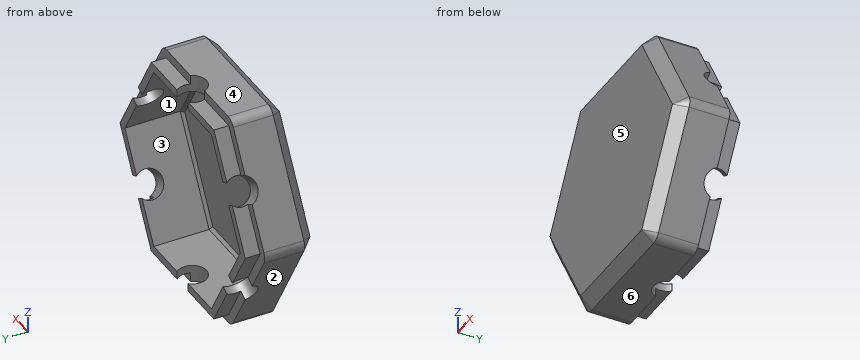
```python
from build123d import *

# Parameters (mm, degrees)
BOSS_EXTRUDE1_START = -3.7
BOSS_EXTRUDE1_DEPTH = 10
CUT_EXTRUDE1_DEPTH  = 8.6
BOSS_EXTRUDE2_DEPTH = 1.6
FILLET1_R           = 2
CUT_EXTRUDE4_DEPTH  = 1
CUT_EXTRUDE3_START  = -3
SKETCH4_R           = 2.5
CUT_EXTRUDE3_DEPTH  = 3
CIRPATTERN1_COUNT   = 6
CHAMFER1_SIZE       = 0.5
CHAMFER2_SIZE       = 2


with BuildPart() as part:
    # Sketch1 → Boss-Extrude1 (new body)
    with BuildSketch(Plane(origin=(0, 0, 0), x_dir=(1, 0, 0), z_dir=(0, 1, 0)).offset(BOSS_EXTRUDE1_START)):
        Polygon((22.5, 0), (11.25, 19.485571585), (-11.25, 19.485571585), (-22.5, 0), (-11.25, -19.485571585), (11.25, -19.485571585), align=None)
    extrude(amount=-BOSS_EXTRUDE1_DEPTH)

    # Sketch2 → Cut-Extrude1 (cut)
    with BuildSketch(Plane(origin=(0, -3.7, 0), x_dir=(1, 0, 0), z_dir=(0, 1, 0))):
        Polygon((-9.517949192, -16.485571585), (9.517949192, -16.485571585), (19.035898385, 0), (9.517949192, 16.485571585), (-9.517949192, 16.485571585), (-19.035898385, 0), align=None)
    extrude(amount=-CUT_EXTRUDE1_DEPTH, mode=Mode.SUBTRACT)

    # Sketch3 → Boss-Extrude2 (add)
    with BuildSketch(Plane(origin=(0, -3.7, 0), x_dir=(1, 0, 0), z_dir=(0, 1, 0))):
        Polygon((10.326239569, -17.885571585), (20.652479139, 0), (10.326239569, 17.885571585), (-10.326239569, 17.885571585), (-20.652479139, 0), (-10.326239569, -17.885571585), align=None)
        Polygon((-9.517949192, -16.485571585), (9.517949192, -16.485571585), (19.035898385, 0), (9.517949192, 16.485571585), (-9.517949192, 16.485571585), (-19.035898385, 0), align=None, mode=Mode.SUBTRACT)
    extrude(amount=BOSS_EXTRUDE2_DEPTH)

    # Fillet1
    fillet1_edges = [part.edges().sort_by_distance(p)[0] for p in [
        (11.25, -8.7, 19.485571585),
        (-11.25, -8.7, 19.485571585),
        (-22.5, -8.7, 0),
        (-11.25, -8.7, -19.485571585),
        (11.25, -8.7, -19.485571585),
        (22.5, -8.7, 0),
    ]]
    fillet(fillet1_edges, radius=FILLET1_R)

    # Sketch6 → Cut-Extrude4 (cut)
    with BuildSketch(Plane(origin=(0, -3.7, 0), x_dir=(1, 0, 0), z_dir=(0, 1, 0))):
        with BuildLine():
            Line((11.827350269, -18.485571585), (21.922649731, -1))
            ThreePointArc((21.922649731, -1), (22.190598923, 0), (21.922649731, 1))
            Line((21.922649731, 1), (11.827350269, 18.485571585))
            ThreePointArc((11.827350269, 18.485571585), (11.095299462, 19.217622393), (10.095299462, 19.485571585))
            Line((10.095299462, 19.485571585), (-10.095299462, 19.485571585))
            ThreePointArc((-10.095299462, 19.485571585), (-11.095299462, 19.217622393), (-11.827350269, 18.485571585))
            Line((-11.827350269, 18.485571585), (-21.922649731, 1))
            ThreePointArc((-21.922649731, 1), (-22.190598923, 0), (-21.922649731, -1))
            Line((-21.922649731, -1), (-11.827350269, -18.485571585))
            ThreePointArc((-11.827350269, -18.485571585), (-11.095299462, -19.217622393), (-10.095299462, -19.485571585))
            Line((-10.095299462, -19.485571585), (10.095299462, -19.485571585))
            ThreePointArc((10.095299462, -19.485571585), (11.095299462, -19.217622393), (11.827350269, -18.485571585))
        make_face()
        Polygon((10.326239569, -17.885571585), (20.652479139, 0), (10.326239569, 17.885571585), (-10.326239569, 17.885571585), (-20.652479139, 0), (-10.326239569, -17.885571585), align=None, mode=Mode.SUBTRACT)
    extrude(amount=-CUT_EXTRUDE4_DEPTH, mode=Mode.SUBTRACT)

    # Sketch4 → Cut-Extrude3 (cut)
    with BuildSketch(Plane(origin=(0, 0, -19.485571585), x_dir=(-1, 0, 0), z_dir=(0, 0, -1)).offset(CUT_EXTRUDE3_START)):
        with Locations((0, -3.8)):
            Circle(SKETCH4_R)
    cut_extrude3 = extrude(amount=CUT_EXTRUDE3_DEPTH, mode=Mode.SUBTRACT)

    # CirPattern1: Cut-Extrude3 ×6 about axis
    cirpattern1_axis = Axis((0, -12.18, 0), (0, 1, 0))
    for i in range(1, CIRPATTERN1_COUNT):
        add(cut_extrude3.rotate(cirpattern1_axis, i * 360 / CIRPATTERN1_COUNT), mode=Mode.SUBTRACT)

    # Chamfer1
    chamfer1_edges = [part.edges().sort_by_distance(p)[0] for p in [
        (0, -12.3, 16.485571585),
        (-14.276923789, -12.3, 8.242785793),
        (-14.276923789, -12.3, -8.242785793),
        (0, -12.3, -16.485571585),
        (14.276923789, -12.3, -8.242785793),
        (14.276923789, -12.3, 8.242785793),
    ]]
    chamfer(chamfer1_edges, length=CHAMFER1_SIZE)

    # Chamfer2
    chamfer2_edges = [part.edges().sort_by_distance(p)[0] for p in [
        (16.875, -13.7, 9.742785793),
        (16.875, -13.7, -9.742785793),
        (0, -13.7, 19.485571585),
        (-16.875, -13.7, 9.742785793),
        (-16.875, -13.7, -9.742785793),
        (0, -13.7, -19.485571585),
        (11.095299462, -13.7, -19.217622393),
        (-11.095299462, -13.7, -19.217622393),
        (-22.190598923, -13.7, 0),
        (-11.095299462, -13.7, 19.217622393),
        (11.095299462, -13.7, 19.217622393),
        (22.190598923, -13.7, 0),
    ]]
    chamfer(chamfer2_edges, length=CHAMFER2_SIZE)


solid = part.part
```
Can you work these out from the model? Positions are in its coordinate system, mm. Face numbers are marked on the shaded views. A direction names the side the tool comes from. Give positions to 0.01 mm unless a question says otherwise; leave off trailing zeros. Order: outer loops, then holes, each group sorted by start corner. A loop starts at its lowest first (then second) coordinate and runs counter-clockwise, first axis right, second up. Notation, with made-up numbers: M -16.5,54 L 41.5,54 A25 cw 41.5,77 Z; hole C 57,-2.5 d4. An arc over 180 degrees is marked long. Write item = value, one per line. Start each with the question number.
Q1. Suppose I cut it at B-B (x = 0). Write out the boundary of the cut face in (y, z), plus the area to 3 significant figures.
Q2. I need wall thicknesses on probe 1 along Z at (x, y) = (0, -8.5); probe 2 along X at (y, z) = (-9.75, -1); probe 3 along Y at (x, z) = (-0.5, -5). Which ranges of each line are inside material? Lowest first, please. Write a range as [from, to].
Q3. Will these pins go through, and if not, where does the flat tip stop? pin 1 Ø16 at (x, z) = (6.5, 2) entering from +Y; pin 2 Ø2 at (y, z) = (-8, 13.5) entering from -X; pin 3 Ø1 at (y, z) = (-5, -3.5) entering from +X.
Q4. Suppose I cut it at A-A (y = -7). Write out the boundary of the cut face in (x, z).
Q5. Suppose I cut it at C-C (z = -14). Write out the boundary of the cut face in (x, y), plus the area to 3 significant figures.
Q6. For the marked faces 1 and 2, which set-ups out of +Z, -Z, +X, -X, +Y, -Y let a thin tool reach every point of the face, with its end or its side?
Q7. We'd pull the mould along Z, two halves only. Please class the marked faces 3, 4, 5 and 6: pulls with the +Z half, pulls with the -Z half, needs draft (parallel to the pull), parting line crosses it, or undercut.
Q8. Suppose I cut it at D-D (x = -6.5). Write out the boundary of the cut face in (y, z).
Check result:
q1.outline = M -13.7,-17.49 L -11.7,-19.49 L -6.3,-19.49 L -6.3,-16.49 L -11.8,-16.49 L -12.3,-15.99 L -12.3,15.99 L -11.8,16.49 L -6.3,16.49 L -6.3,19.49 L -11.7,19.49 L -13.7,17.49 Z
q1.area = 86.8 mm2
q2.probe_1 = [-19.49, -16.49], [16.49, 19.49]
q2.probe_2 = [-21.92, -18.46], [18.46, 21.92]
q2.probe_3 = [-13.7, -12.3]
q3.pin_1 = -12.3
q3.pin_2 = -15.28
q3.pin_3 = 20.77
q4.outline = M -21.92,-1 L -11.83,-18.49 A2 ccw -10.1,-19.49 L 10.1,-19.49 A2 ccw 11.83,-18.49 L 21.92,-1 A2 ccw 21.92,1 L 11.83,18.49 A2 ccw 10.1,19.49 L -10.1,19.49 A2 ccw -11.83,18.49 L -21.92,1 A2 ccw Z; hole M -19.04,0 L -9.52,-16.49 L 9.52,-16.49 L 19.04,0 L 9.52,16.49 L -9.52,16.49 Z
q5.outline = M -14.42,-11.7 L -12.11,-13.7 L 12.11,-13.7 L 14.42,-11.7 L 14.42,-4.7 L 12.57,-4.7 L 12.57,-2.1 L 10.95,-2.1 L 10.95,-11.8 L 10.38,-12.3 L -10.38,-12.3 L -10.95,-11.8 L -10.95,-2.1 L -12.57,-2.1 L -12.57,-4.7 L -14.42,-4.7 Z
q5.area = 97.1 mm2
q6.face_1 = +Y
q6.face_2 = -Z, -X, +Y, -Y
q7.face_3 = undercut
q7.face_4 = pulls with the +Z half
q7.face_5 = needs draft
q7.face_6 = pulls with the -Z half
q8.outline = M -13.7,-17.49 L -11.7,-19.49 L -4.7,-19.49 L -4.7,-17.89 L -2.1,-17.89 L -2.1,-16.49 L -11.8,-16.49 L -12.3,-15.99 L -12.3,15.99 L -11.8,16.49 L -2.1,16.49 L -2.1,17.89 L -4.7,17.89 L -4.7,19.49 L -11.7,19.49 L -13.7,17.49 Z
